```python
from build123d import *

# Parameters (mm, degrees)
F0_W     = 266.7
F0_H     = 165.1
F1_DEPTH = 165.1
F2_W     = 241.3
F2_H     = 152.4
F3_DEPTH = 152.4
F4_W     = 12.7
F4_H     = 12.7
F5_DEPTH = 152.4


with BuildPart() as f1:
    # F0 (on Front) → F1 (new body)
    with BuildSketch(Plane.XZ):
        with Locations((-17.048836, -1.777712)):
            Rectangle(F0_W, F0_H)
    extrude(amount=-F1_DEPTH)

    # F2 (on face) → F3 (cut)
    with BuildSketch(Plane.XZ):
        with Locations((-17.048836, -1.777712)):
            Rectangle(F2_W, F2_H)
    extrude(amount=-F3_DEPTH, mode=Mode.SUBTRACT)

    # F4 (on face) → F5 (cut)
    with BuildSketch(Plane.XZ):
        with Locations((-144.048836, -52.577712)):
            Rectangle(F4_W, F4_H)
        with Locations((-144.048836, -1.777712)):
            Rectangle(F4_W, F4_H)
        with Locations((-144.048836, 49.022288)):
            Rectangle(F4_W, F4_H)
        with Locations((109.951164, -52.577712)):
            Rectangle(F4_W, F4_H)
        with Locations((109.951164, -1.777712)):
            Rectangle(F4_W, F4_H)
        with Locations((109.951164, 49.022288)):
            Rectangle(F4_W, F4_H)
    extrude(amount=-F5_DEPTH, mode=Mode.SUBTRACT)


solid = f1.part
```
Source: CAD feature listing. Evaluate the final solid. Frame: model axes, mm. A direction names the side the tool comes from. Coordinates: 2 decimals unless noted, no trailing zeros. Loops run counter-clockwise (first coordinate to the right, second up) from the corner with the lowest first, then second, coordinate; pieces in that order, holes last. Notation, with made-up numbers: M -33,-29 L -19,-29 A17 ccw -19,-7 Z; hole C 52.25,72.25 d4. An arc over 180 degrees is marked long. Put each result on its own line as item: value. Start each with the question number.
1) Cut plane C-C on x = -11. Return the cut outline in (y, z).
2) Ray query, L1, parallel to Z at x = -97, y = 27.5; L2, parallel to X at y = 86, z = -35.5; L3, parallel to Y at x = -30.5, z = -52. Return the intervals inside material, ascending. Write a range as from..to.
3) Cut plane B-B on z = -33.5. Return the cut outline in (x, y), then the cut area to 3 significant figures.
4) Pull-direction query (X, two-part tool) for faces 1 (the face through (-19, 75, -77.978)), 2 (the face through (-144, 75, -46.228)), 3 (the face through (-150.399, 81, -21)); classes: pulls with the +X half, pulls with the -X half, needs draft (parallel to the pull), parting line crosses it, or undercut.
5) Reachability of faces 4 (the face through (-144, 0, -27)), 5 (the face through (-19, 75, 74.422)), 6 (the face through (-144, 75, 42.672)) from +Z, -Z, +X, -X, +Y, -Y: full face, straight path, thin tool, end or side. Return the list, or none.
6) Cut plane A-A on y = 149.5. Give the number of separate pieces and of enclosed holes in the cut face, then the cut area to 3 significant figures.
The answers:
1. outline: M 0,-84.33 L 165.1,-84.33 L 165.1,80.77 L 0,80.77 L 0,74.42 L 152.4,74.42 L 152.4,-77.98 L 0,-77.98 Z
2. L1: z = -84.33..-77.98, 74.42..80.77
2. L2: x = -150.4..-137.7, 103.6..116.3
2. L3: y = 152.4..165.1
3. outline: M -150.4,0 L -137.7,0 L -137.7,152.4 L 103.6,152.4 L 103.6,0 L 116.3,0 L 116.3,165.1 L -150.4,165.1 Z
3. area: 7,260 mm²
4. face 1: undercut
4. face 2: needs draft
4. face 3: pulls with the -X half
5. face 4: +Z, -Z, +X, -X, -Y
5. face 5: -Y
5. face 6: +X, -X, -Y
6. separate pieces: 6
6. enclosed holes: 0
6. area: 6,290 mm²
